```python
from build123d import *

# Parameters (mm, degrees)
SKETCH_1_R          = 50
EXTRUDE_1_DEPTH     = 20
FILLET_1_R          = 5
SKETCH_2_R          = 7.5
CUT_EXTRUDE_1_DEPTH = 30


with BuildPart() as part:
    # 草图1 → 凸台-拉伸1 (new body)
    with BuildSketch(Plane(origin=(0, 0, 0), x_dir=(0, 0, -1), z_dir=(1, 0, 0))):
        Circle(SKETCH_1_R)
    extrude(amount=EXTRUDE_1_DEPTH)

    # 圆角1
    fillet_1_edges = [part.edges().sort_by_distance(p)[0] for p in [
        (0, 0, 50),
        (20, 0, 50),
    ]]
    fillet(fillet_1_edges, radius=FILLET_1_R)

    # 草图2 → 切除-拉伸1 (cut)
    with BuildSketch(Plane.ZY):
        Circle(SKETCH_2_R)
    extrude(amount=-CUT_EXTRUDE_1_DEPTH, mode=Mode.SUBTRACT)


solid = part.part
```
Work out the finished part from the listing and answer in its coordinate system (mm). Round coordinates to 2 decimals unless told otherwise and drop trailing zeros. Write each loop counter-clockwise with the first axis right and the second up, starting at its lowest first coordinate (ties: lowest second). Pieces come first, ordered by that corner, then holes. Notation, with made-up numbers: (76.25, -3) -> (82.25, -3) arc R21 cw to (82.25, 8) -> close; hole circle Ø1 at (30, 21). An arc over 180 degrees is marked (long way). Write each question's results on one line, items separated by ' | '.
1) For a pull along Z with two mould halves and no side action, classify faces 1 (the cylindrical face through (9.93, 15.02, -47.69)), 2 (the flat face through (20, -9, 1)), 3 (the cylindrical face through (9.86, 0.33, -7.493)) as +Z half, -Z half, draft (parallel to the pull), parting line (faces both ways), or undercut.
Findings:
face 1: parting line | face 2: draft | face 3: undercut
2) Consider line 1 along Y through (x, z) = (5.25, 0); line 2 along Y through (x, z) = (13.5, 6); line 3 along Z through (x, y) = (2.25, 33.5). Determine where each line is inside the solid, lowest interval first. Write a range as [from, to].
Findings:
line 1: y = [-50, -7.5], [7.5, 50] | line 2: y = [-49.64, -4.5], [4.5, 49.64] | line 3: z = [-36, 36]
3) Flat-ended cylindrical pins translate along their axes: pin 1 (2 mm diameter, centred on x = 16, z = -5.5, fed in from +Y); pin 2 (4 mm diameter, centred on x = 12, y = 32, fed in from +Z); pin 3 (12 mm diameter, centred on x = 2, y = 23, fed in from +Z). Find the tip coordinate at first contact, or state that the pin passes through.
Findings:
pin 1: stops at y = 49.76 | pin 2: stops at z = 40 | pin 3: stops at z = 46.8
4) The part is cut by section A-A (z = 0). Write down the section's boundary in (x, y).
Findings:
outline: (0, -45) arc R5 ccw to (5, -50) -> (15, -50) arc R5 ccw to (20, -45) -> (20, -7.5) -> (0, -7.5) -> close; (0, 7.5) -> (20, 7.5) -> (20, 45) arc R5 ccw to (15, 50) -> (5, 50) arc R5 ccw to (0, 45) -> close
5) The part is cut by section C-C (x = 17). Write down the section's boundary in (y, z), and give its area (3 significant figures).
Findings:
outline: circle Ø99.17 at (0, 0); hole circle Ø15 at (0, 0) | area: 7,550 mm²
